Geometry: final body of the model. Coordinates: model frame, mm. A direction names the side the tool comes from. Coordinates: 2 decimals unless noted, no trailing zeros. Write each loop counter-clockwise with the first axis right and the second up, starting at its lowest first coordinate (ties: lowest second). Pieces come first, ordered by that corner, then holes. Notation, with made-up numbers: M 16.25,-29 L 43.25,-29 A22 ccw 43.25,-10 Z; hole C -22,-29.5 d9. An arc over 180 degrees is marked long. Write item = value, one per line. Start each with the question number.
Item 1: Ray query, L1, parallel to Z at x = 91, y = -8.5; L2, parallel to Z at x = -50.5, y = 1.5; L3, parallel to X at y = 7.25, z = -8. Return the intervals inside material, ascending. Write a range as [from, to].
Item 2: Section C-C on z = 83. Output: boundary loops of the cut face in (x, y).
Item 3: First-contact query: pin 1 Ø4 at (y, z) = (-1, 44) entering from -X; pin 2 Ø12 at (x, y) = (72.5, -6) entering from +Z; pin 3 Ø2 at (y, z) = (7.5, 69) entering from -X. Flat tips, straight axial feed; report the tip coordinate or a pass-through.
Item 4: Reachability of faces 1 (the cylindrical face through (4.38, -8.43, 112.1)), 2 (the flat face through (-1, -12.5, 1)) from +Z, -Z, +X, -X, +Y, -Y: full face, straight path, thin tool, end or side. Return the list, or none.
Item 5: Section A-A on x = 0. Output: boundary loops of the cut face in (y, z), plus the area to 4 significant figures.
Item 6: Section B-B on y = 0. Output: boundary loops of the cut face in (x, z).
from build123d import *

# Parameters (mm, degrees)
F0_R      = 100
F1_DEPTH  = 12.5
F1_FACE_R = 100
F2_DEPTH  = 12.5
F3_R      = 9.5
F4_DEPTH  = 125


with BuildPart() as f1:
    # F0 (on Front) → F1 (new body)
    with BuildSketch(Plane.XZ):
        Circle(F0_R)
    extrude(amount=F1_DEPTH)

    # F1_face (on face) → F2 (join)
    with BuildSketch(Plane(origin=(0, 0, 0), x_dir=(1, 0, 0), z_dir=(0, 1, 0))):
        Circle(F1_FACE_R)
    extrude(amount=F2_DEPTH)

    # F3 (on Top) → F4 (join)
    with BuildSketch(Plane.XY):
        Circle(F3_R)
    extrude(amount=F4_DEPTH)


solid = f1.part
Responses:
q1.L1 = [-41.46, 41.46]
q1.L2 = [-86.31, 86.31]
q1.L3 = [-99.68, 99.68]
q2.outline = M -55.78,-12.5 L 55.78,-12.5 L 55.78,12.5 L -55.78,12.5 Z
q3.pin_1 = -90.75
q3.pin_2 = 74.68
q3.pin_3 = -73.32
q4.face_1 = +Z
q4.face_2 = +Z, -Z, +X, -X, -Y
q5.outline = M -12.5,-100 L 12.5,-100 L 12.5,100 L 9.5,100 L 9.5,125 L -9.5,125 L -9.5,100 L -12.5,100 Z
q5.area = 5,475 mm²
q6.outline = M -9.5,99.55 A100 ccw long 9.5,99.55 L 9.5,125 L -9.5,125 Z
